Read the model definition and answer for the solid it produces. Units are mm, in the model's axes. Face numbers are marked on the shaded views. A direction names the side the tool comes from. Give positions to 0.01 mm unless a question says otherwise; leave off trailing zeros. Loops run counter-clockwise (first coordinate to the right, second up) from the corner with the lowest first, then second, coordinate; pieces in that order, holes last. Notation, with made-up numbers: (33, -16.75) - (48, -16.75) arc R22 ccw to (48, 16.25) - close; hole circle Ø1 at (-7, 69.25). An arc over 180 degrees is marked (long way). Use a Markdown table: item, result. Add a question column.
Item 1: For a pull along Y with two mould halves and no side action, classify the marked faces 1, 2, 3 and 4 as +Y half, -Y half, draft (parallel to the pull), parting line (faces both ways), or undercut.
Item 2: A cutting plane is placed at B-B (x = 2). Give the number of separate pieces and of enclosed holes in the cut face, plus the area to 3 significant figures.
Item 3: Each of these flat-tipped pins is pushed along its axis until it touches: P1, Ø3, axis at x = 4, y = 34.5, coming from the -Z side; P2, Ø3, axis at x = 4.5, z = -3, coming from the -Y side; P3, Ø7.5, axis at y = 46.83, z = 25.4, coming from the -X side; P4, Ø3, axis at x = 5.5, z = -3.5, coming from the +Y side. Where does it stop, or does it pass through?
Item 4: Which of the six approach directions +Z, -Z, +X, -X, +Y, -Y give full straight-line access (tool end or side, diameter ignored) to the marked faces 5 and 6?
Item 5: A cutting plane is placed at A-A (z = 25.4). Determine the outline of the cut face in (x, y) (3 decimals), plus the area to 3 significant figures.
Item 6: Consider probe 1 along Y at (x, z) = (5.75, 25.4); probe 2 along Y at (x, z) = (2.75, 24); probe 3 along Z at (x, y) = (3.75, 22). Determine where each line is inside the solid, lowest interval first. Write a range as [from, to].
Item 7: A cutting plane is placed at C-C (y = 20). Determine the outline of the cut face in (x, z) (3 decimals), plus the area to 3 significant figures.
from build123d import *

# Parameters (mm, degrees)
SKETCH1_W           = 76.2
SKETCH1_H           = 50.8
BOSS_EXTRUDE1_DEPTH = 9.525
SKETCH3_R           = 3.175
SKETCH3_R_2         = 4.7625
CUT_EXTRUDE1_DEPTH  = 93.075
SKETCH4_W           = 9.525
SKETCH4_H           = 12.7
BOSS_EXTRUDE2_DEPTH = 6.35


with BuildPart() as part:
    # Sketch1 → Boss-Extrude1 (new body)
    with BuildSketch(Plane.YZ):
        with Locations((38.1, 25.4)):
            Rectangle(SKETCH1_W, SKETCH1_H)
    extrude(amount=BOSS_EXTRUDE1_DEPTH)

    # Sketch3 → Cut-Extrude1 (cut, through all)
    with BuildSketch(Plane.YZ.offset(9.525)):
        with Locations(Location((29.36875, 25.4, 0), (0, 0, 270))):
            Circle(SKETCH3_R)
        with Locations(Location((46.83125, 25.4, 0), (0, 0, 270))):
            Circle(SKETCH3_R_2)
    extrude(amount=-CUT_EXTRUDE1_DEPTH, mode=Mode.SUBTRACT)

    # Sketch4 → Boss-Extrude2 (add)
    with BuildSketch(Plane(origin=(0, 0, 0), x_dir=(1, 0, 0), z_dir=(0, 0, -1))):
        with Locations((4.7625, -12.7)):
            Rectangle(SKETCH4_W, SKETCH4_H)
        with Locations((4.7625, -63.5)):
            Rectangle(SKETCH4_W, SKETCH4_H)
    extrude(amount=BOSS_EXTRUDE2_DEPTH)


solid = part.part
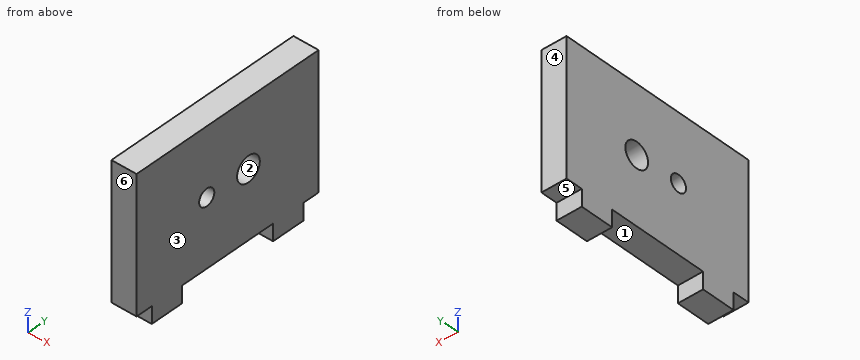
Geometry says:
| question | item | result |
|---|---|---|
| 1 | face 1 | undercut |
| 1 | face 2 | undercut |
| 1 | face 3 | draft |
| 1 | face 4 | +Y half |
| 2 | separate pieces | 1 |
| 2 | enclosed holes | 2 |
| 2 | area | 3,930 mm² |
| 3 | P1 | z = 0 |
| 3 | P2 | y = 6.35 |
| 3 | P3 | through |
| 3 | P4 | y = 69.85 |
| 4 | face 5 | -Z, +X, -X, +Y |
| 4 | face 6 | +Z, -Z, +X, -X, -Y |
| 5 | outline | (0, 0) - (9.525, 0) - (9.525, 26.194) - (0, 26.194) - close; (0, 32.544) - (9.525, 32.544) - (9.525, 42.069) - (0, 42.069) - close; (0, 51.594) - (9.525, 51.594) - (9.525, 76.2) - (0, 76.2) - close |
| 5 | area | 575 mm² |
| 6 | probe 1 | [0, 26.19], [32.54, 42.07], [51.59, 76.2] |
| 6 | probe 2 | [0, 26.52], [32.22, 42.28], [51.38, 76.2] |
| 6 | probe 3 | [0, 50.8] |
| 7 | outline | (0, 0) - (9.525, 0) - (9.525, 50.8) - (0, 50.8) - close |
| 7 | area | 484 mm² |
